Check sheet for the modelled part. Datum: model origin and axes. Units: mm. Round coordinates to 2 decimals unless told otherwise and drop trailing zeros. Write each loop counter-clockwise with the first axis right and the second up, starting at its lowest first coordinate (ties: lowest second). Pieces come first, ordered by that corner, then holes. Notation, with made-up numbers: M 26.5,49 L 68.5,49 A22 ccw 68.5,71 Z; hole C -34,-36 d10. An arc over 180 degrees is marked long. Answer in a Markdown table with one row per item.
```python
from build123d import *

# Parameters (mm, degrees)
SKETCH1_R           = 5.650668072
SKETCH1_R_2         = 1.75
BOSS_EXTRUDE1_DEPTH = 2.8
FILLET1_R           = 2


with BuildPart() as part:
    # Sketch1 → Boss-Extrude1 (new body)
    with BuildSketch(Plane.XY):
        Polygon((11.547005384, 20), (27.5, 0), (11.547005384, -20), (-11.547005384, -20), (-27.5, 0), (-11.547005384, 20), align=None)
        Circle(SKETCH1_R, mode=Mode.SUBTRACT)
        with Locations((-24.25, 0)):
            Circle(SKETCH1_R_2, mode=Mode.SUBTRACT)
        with Locations((24.25, 0)):
            Circle(SKETCH1_R_2, mode=Mode.SUBTRACT)
    extrude(amount=BOSS_EXTRUDE1_DEPTH)

    # Fillet1
    fillet1_edges = [part.edges().sort_by_distance(p)[0] for p in [
        (27.5, 0, 1.4),
        (-27.5, 0, 1.4),
    ]]
    fillet(fillet1_edges, radius=FILLET1_R)


solid = part.part
```
1. Section check B-B, the plane x = 0. Record the cut outline in (y, z).
Found:
| item | result |
|---|---|
| outline | M -20,0 L -5.65,0 L -5.65,2.8 L -20,2.8 Z; M 5.65,0 L 20,0 L 20,2.8 L 5.65,2.8 Z |
2. Go/stop test with a flat-tipped pin: pin 1 (8 mm diameter, centred on x = -3, y = -8, fed in from -Z). Record where the tip stops, or that it passes through.
Found:
| item | result |
|---|---|
| pin 1 | stops at z = 0 |
3. Draft check along X on faces 1 (the face through (-18.921, -10.755, 1.38)), 2 (the face through (0, 20, 1)), 3 (the face through (22.5, 0.08, 1.38)). Enter one of: +X half, -X half, draft (parallel to the pull), parting line (faces both ways), or undercut.
Found:
| item | result |
|---|---|
| face 1 | -X half |
| face 2 | draft |
| face 3 | undercut |
4. Scan lines: L1, parallel to Y at x = 0, z = 2.15; L2, parallel to Y at x = -2, z = 0.5; L3, parallel to X at y = -4.5, z = 2.5. Record each from-to range of solid material in increasing order.
Found:
| item | result |
|---|---|
| L1 | y = -20 to -5.65, 5.65 to 20 |
| L2 | y = -20 to -5.28, 5.28 to 20 |
| L3 | x = -23.91 to -3.42, 3.42 to 23.91 |
5. Section check D-D, the plane y = -10.5. Record the cut outline in (x, z), and give its area (3 significant figures).
Found:
| item | result |
|---|---|
| outline | M -19.12,0 L 19.12,0 L 19.12,2.8 L -19.12,2.8 Z |
| area | 107 mm2 |
6. Section check C-C, the plane x = 24.25. Record the cut outline in (y, z).
Found:
| item | result |
|---|---|
| outline | M -4.07,0 L -1.75,0 L -1.75,2.8 L -4.07,2.8 Z; M 1.75,0 L 4.07,0 L 4.07,2.8 L 1.75,2.8 Z |
7. Section check A-A, the plane y = 0. Record the cut outline in (x, z), and give its area (3 significant figures).
Found:
| item | result |
|---|---|
| outline | M -26.94,0 L -26,0 L -26,2.8 L -26.94,2.8 Z; M -22.5,0 L -5.65,0 L -5.65,2.8 L -22.5,2.8 Z; M 5.65,0 L 22.5,0 L 22.5,2.8 L 5.65,2.8 Z; M 26,0 L 26.94,0 L 26.94,2.8 L 26,2.8 Z |
| area | 99.6 mm2 |
